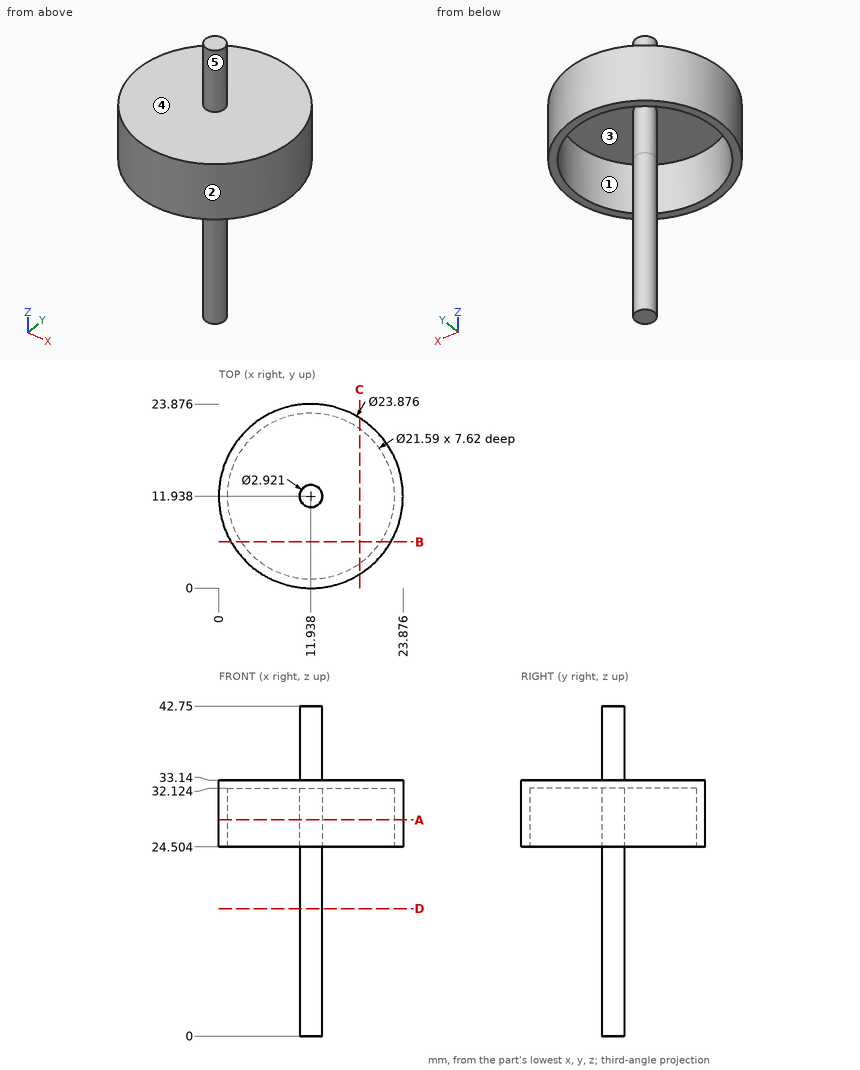
Here's the drawing with two shaded views (mm, measured from the low corner). I have some questions. A direction names the side the tool comes from. Round coordinates to 2 decimals unless told otherwise and drop trailing zeros. Loops run counter-clockwise (first coordinate to the right, second up) from the corner with the lowest first, then second, coordinate; pieces in that order, holes last. Notation, with made-up numbers: (62.25, -32.75) -> (72.25, -32.75) arc R13 ccw to (72.25, -25.75) -> close; hole circle Ø9 at (76, 33.25). An arc over 180 degrees is marked (long way). Answer as CSV lines item,"result". Start each with the question number.
1. For the marked faces 1 and 2, which set-ups out of +Z, -Z, +X, -X, +Y, -Y let a thin tool reach every point of the face, with its end or its side?
2. Imagine slicing it at A-A on z = 28. Write out the boundary of the cut face in (x, y) (1 decimal).
3. If we mould it in two halves opening along X, with no side actions, what happens to the marked faces 3, 4 and 5? For each: pulls with the +X half, pulls with the -X half, needs draft (parallel to the pull), parting line crosses it, or undercut.
4. Imagine slicing it at B-B on y = 6. Write out the boundary of the cut face in (x, z).
5. Imagine slicing it at C-C on x = 18.25. Write out the boundary of the cut face in (y, z), plus the area to 3 significant figures.
6. I need wall thicknesses on probe 1 along Z at (x, y) = (22.25, 10.25); probe 2 along Z at (x, y) = (19.5, 20.5); probe 3 along Y at (x, z) = (12.25, 30). Which ranges of each line are inside material? Lowest first, please. Write a range as from..to.
7. Imagine slicing it at D-D on z = 16.5. Write out the boundary of the cut face in (x, y).
8. I'm going to push flat-ended pins straight in: P1, Ø1.5, axis at y = 10, z = 20, coming from the +X side; P2, Ø4, axis at x = 9.5, y = 4.5, coming from the +Z side; P3, Ø12, axis at x = 13, z = 12.5, coming from the +Y side. Where does each tip first touch, or does it pass through?
Solution:
1,face 1,"-Z"
1,face 2,"+Z, -Z"
2,outline,"circle Ø23.9 at (11.9, 11.9); circle Ø2.9 at (11.9, 11.9); hole circle Ø21.6 at (11.9, 11.9)"
3,face 3,"undercut"
3,face 4,"needs draft"
3,face 5,"parting line crosses it"
4,outline,"(1.58, 24.5) -> (2.92, 24.5) -> (2.92, 32.12) -> (20.95, 32.12) -> (20.95, 24.5) -> (22.29, 24.5) -> (22.29, 33.14) -> (1.58, 33.14) -> close"
5,outline,"(1.81, 24.5) -> (3.18, 24.5) -> (3.18, 32.12) -> (20.7, 32.12) -> (20.7, 24.5) -> (22.07, 24.5) -> (22.07, 33.14) -> (1.81, 33.14) -> close"
5,area,"41.6 mm²"
6,probe 1,"32.12..33.14"
6,probe 2,"24.5..33.14"
6,probe 3,"0..1.15, 10.51..13.36, 22.73..23.87"
7,outline,"circle Ø2.92 at (11.94, 11.94)"
8,P1,"x = 12.79"
8,P2,"z = 33.14"
8,P3,"y = 13.4"
